```python
from build123d import *

# Parameters (mm, degrees)
BOSS_EXTRUDE1_DEPTH = 1.1116
SKETCH2_R           = 5.0292
BOSS_EXTRUDE2_DEPTH = 1.1684
BOSS_EXTRUDE3_DEPTH = 96.52
SKETCH4_W           = 6.35
SKETCH4_H           = 7.496
CHAMFER1_SIZE       = 1
SKETCH5_R           = 3.175
CUT_EXTRUDE1_DEPTH  = 9.525


with BuildPart() as part:
    # Sketch1 → Boss-Extrude1 (new body)
    with BuildSketch(Plane(origin=(0, 0, -68.704), x_dir=(-1, 0, 0), z_dir=(0, 0, -1))):
        Polygon((-3.666174209, 6.35), (-7.332348419, 0), (-3.666174209, -6.35), (3.666174209, -6.35), (7.332348419, 0), (3.666174209, 6.35), align=None)
    extrude(amount=-BOSS_EXTRUDE1_DEPTH)

    # Sketch2 → Boss-Extrude2 (add)
    with BuildSketch(Plane.XY.offset(-67.5924)):
        Circle(SKETCH2_R)
    extrude(amount=BOSS_EXTRUDE2_DEPTH)

    # Sketch3 → Boss-Extrude3 (add)
    with BuildSketch(Plane(origin=(0, 0, -66.424), x_dir=(-1, 0, 0), z_dir=(0, 0, -1))):
        Polygon((3.666174209, -6.35), (7.332348419, 0), (3.666174209, 6.35), (-3.666174209, 6.35), (-7.332348419, 0), (-3.666174209, -6.35), align=None)
    extrude(amount=-BOSS_EXTRUDE3_DEPTH)

    # Sketch4 → Revolve1 (revolve)
    with BuildSketch(Plane.XZ, mode=Mode.PRIVATE) as revolve1_sk:
        with Locations((3.175, -72.452)):
            Rectangle(SKETCH4_W, SKETCH4_H)
    revolve(revolve1_sk.sketch.rotate(Axis((0, 0, -68.704), (0, 0, -1)), 180), axis=Axis((0, 0, -68.704), (0, 0, -1)))

    # Chamfer1
    chamfer1_edges = [part.edges().sort_by_distance(p)[0] for p in [
        (6.35, 0, -76.2),
    ]]
    chamfer(chamfer1_edges, length=CHAMFER1_SIZE)

    # Sketch5 → Cut-Extrude1 (cut)
    with BuildSketch(Plane.XY.offset(30.096)):
        Circle(SKETCH5_R)
    extrude(amount=-CUT_EXTRUDE1_DEPTH, mode=Mode.SUBTRACT)


solid = part.part
```
The model under review builds one solid part; all positions refer to its coordinate system, in mm. A direction names the side the tool comes from. Round coordinates to 2 decimals unless told otherwise and drop trailing zeros. Order: outer loops, then holes, each group sorted by start corner. A loop starts at its lowest first (then second) coordinate and runs counter-clockwise, first axis right, second up.
Item 1: Add section A-A, the plane z = -22.5. State the section outline as (x, y) points, and give its area (3 significant figures).
Working result:
outline: (-7.33, 0) - (-3.67, -6.35) - (3.67, -6.35) - (7.33, 0) - (3.67, 6.35) - (-3.67, 6.35) - close
area: 140 mm2
Item 2: For pin 1 (6 mm diameter, centred on y = 4, z = -15.5, fed in from +X) (3 decimals); pin 2 (1 mm diameter, centred on y = 4.5, z = -61.5, fed in from +X), all flat-tipped, find the tip position at first contact; note any pin that passes through.
Working result:
pin 1: stops at x = 6.755
pin 2: stops at x = 5.02
Item 3: To check wall thickness, follow probe 1 along Y at (x, z) = (0, 24) (3 decimals); probe 2 along Z at (x, y) = (0.25, -1.75); probe 3 along Y at (x, z) = (-5.5, -27). State the ranges of each line that lie inside material, in increasing order.
Working result:
probe 1: y = -6.35 to -3.175, 3.175 to 6.35
probe 2: z = -76.2 to 20.57
probe 3: y = -3.17 to 3.17
Item 4: Draft analysis for pull direction Y (two halves, no side actions). For faces 4 (the flat face through (7, 0, -68.704)), 5 (the flat face through (0, -6.35, -19)), 6 (the flat face through (0, 0, 20.571)), state which applies: released by +Y, released by -Y, zero draft, split by the parting line, or undercut.
Working result:
face 4: zero draft
face 5: released by -Y
face 6: undercut
Item 5: Machinability: for faces 1 (the cylindrical face through (-0.69, -3.1, 25.4)), 2 (the cylindrical face through (-1.09, -4.91, -67.02)), 3 (the cylindrical face through (-2.93, -5.634, -71.907)), which of the approach directions +Z, -Z, +X, -X, +Y, -Y give a long, thin tool a straight path to every point of the face, cutting with its end or side? Answer none if there is none.
Working result:
face 1: +Z
face 2: none
face 3: -Z
